Answer from the drawing. Dimensions are ordinates in mm from the lowest x, y and z of the part. A direction names the side the tool comes from. Coordinates: 2 decimals unless noted, no trailing zeros. Write each loop counter-clockwise with the first axis right and the second up, starting at its lowest first coordinate (ties: lowest second). Pieces come first, ordered by that corner, then holes. Notation, with made-up numbers: (-15.5, 57.25) - (34.5, 57.25) arc R24 cw to (34.5, 83.25) - close; hole circle Ø4 at (84.25, 53.25). An arc over 180 degrees is marked (long way). Return JSON: item names as keys, results as strings.
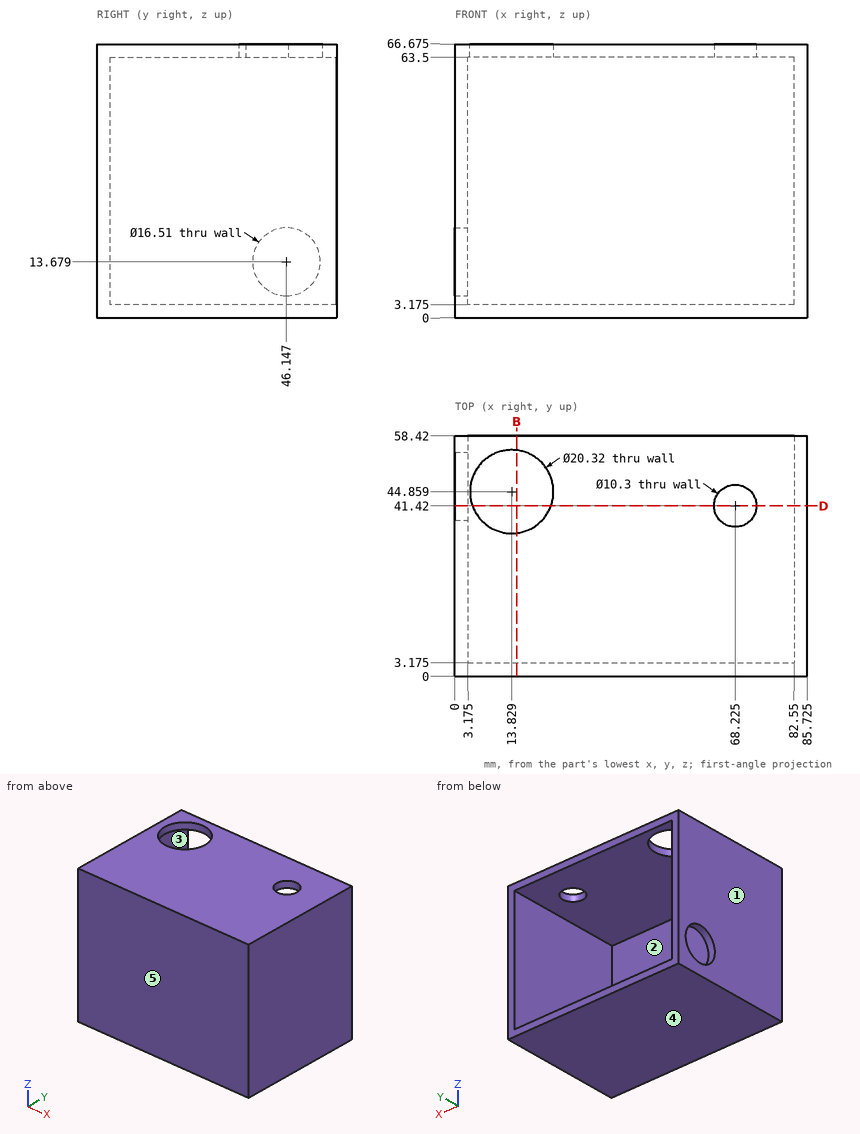
(1) Determine the mould class of the marked faces 3, 4 and 5 for opening direction Z: +Z half, -Z half, draft (parallel to the pull), parting line (faces both ways), or undercut.
Answer:
{"face 3": "undercut", "face 4": "-Z half", "face 5": "draft"}
(2) A cutting plane is placed at B-B (x = 15). Determine the outline of the cut face in (y, z) (1 decimal).
Answer:
{"outline": "(0, 0) - (58.4, 0) - (58.4, 3.2) - (3.2, 3.2) - (3.2, 63.5) - (34.8, 63.5) - (34.8, 66.7) - (0, 66.7) - close; (55, 63.5) - (58.4, 63.5) - (58.4, 66.7) - (55, 66.7) - close"}
(3) Flat-ended cylindrical pins translate along their axes: P1, Ø10, axis at y = 46.15, z = 13.68, coming from the -X side; P2, Ø10, axis at x = 73.5, z = 54.5, coming from the +Y side (3 decimals). Find the tip coordinate at first contact, or state that the pin passes through.
Answer:
{"P1": "x = 82.55", "P2": "y = 3.175"}
(4) A cutting plane is placed at D-D (y = 41.42). State how many separate pieces and enclosed holes the cut face has, and give its area (3 significant figures).
Answer:
{"separate pieces": "3", "enclosed holes": "0", "area": "791 mm²"}
(5) Straight lines are drawn through the part: line 1 (Z direction, x = 66.5, y = 16.5) (1 decimal); line 2 (Y direction, x = 28.5, z = 60.5) (1 decimal). For each, find the intervals that lie inside material, in ascending order. Write a range as from..to.
Answer:
{"line 1": "0..3.2, 63.5..66.7", "line 2": "0..3.2"}
(6) Which of the six approach directions +Z, -Z, +X, -X, +Y, -Y give full straight-line access (tool end or side, diameter ignored) to the marked faces 1 and 2?
Answer:
{"face 1": "+Z, -Z, -X, +Y, -Y", "face 2": "+Y"}
